Autodesk Inventor part; units mm, degrees
ref_plane "YZ Plane" through (0, 0, 0) normal (1, 0, 0) x (0, 1, 0)
ref_plane "XZ Plane" through (0, 0, 0) normal (0, 1, 0) x (-1, 0, 0)
ref_plane "XY Plane" through (0, 0, 0) normal (0, 0, 1) x (1, 0, 0)
sketch "スケッチ1" plane through (0, 0, 0) normal (0, 0, 1) x (1, 0, 0)
  circle A0 centre (0, 0) radius 1.5
  dimension "d0" = 3
extrude "押し出し1" add sketch "スケッチ1" along normal blind 6
sketch "スケッチ2" plane through (0, 0, 6) normal (0, 0, 1) x (1, 0, 0)
  circle A0 centre (0, 0) radius 1.5
  circle A1 centre (0, 0) radius 3
  dimension "d3" = 6
extrude "押し出し2" add sketch "スケッチ2" along normal blind 2 contours A0 | A1
fillet "フィレット1" radius 2 1 edges at (-3, 0, 8)
thread "ねじ1"
sketch "スケッチ3" plane through (0, 0, 0) normal (0, 0, -1) x (-1, 0, 0)
  circle A0 centre (0, 0) radius 1.5
extrude "押し出し3" add sketch "スケッチ3" along normal blind 9
sketch "スケッチ4" plane through (0, 0, -9) normal (0, 0, -1) x (-1, 0, 0)
  circle A0 centre (0, 0) radius 1.5
extrude "押し出し4" add sketch "スケッチ4" along normal blind 7
properties part number "SB　22mmなべネジ" material "Steel, Mild"
The model under review builds one solid part; all positions refer to its coordinate system, in mm. A direction names the side the tool comes from. Give positions to 0.01 mm unless a question says otherwise; leave off trailing zeros. Loops run counter-clockwise (first coordinate to the right, second up) from the corner with the lowest first, then second, coordinate; pieces in that order, holes last. Notation, with made-up numbers: (83.25, 38) -> (136.25, 38) arc R10 ccw to (136.25, 42) -> close; hole circle Ø11 at (55, -5.75). An arc over 180 degrees is marked (long way). Answer as a JSON object with one key per item and string values. Group by question number.
Q1. Wall thickness on line 1 along Z through (x, y) = (-0.5, 1); line 2 along X through (y, z) = (0, 1.25): over which ranges is each line inside the solid? List them lowest first.
Q2. Tool access review of faces 1 (the flat face through (1.3, -1.3, 6)), 2 (the flat face through (0, 0, -16)): name each direction out of +Z, -Z, +X, -X, +Y, -Y from which nothing blocks a thin tool from reaching the whole face with its end or side.
Q3. Insertion check: pin 1 (3 mm diameter, centred on y = 0.5, z = -9.5, fed in from -X); pin 2 (1.5 mm diameter, centred on x = 2.5, y = -1, fed in from +Z); pin 3 (1 mm diameter, centred on x = -1.5, y = 0, fed in from +Z). Each pin has a flat end and moves straight along its axis. Give the tip position at first contact, or say it passes through.
Q4. Take a section at A-A (z = -5). Write out the cut boundary in (x, y).
Answer below:
{
 "1": {"line 1": "z = -16 to 8", "line 2": "x = -1.5 to 1.5"},
 "2": {"face 1": "-Z", "face 2": "-Z, +X, -X, +Y, -Y"},
 "3": {"pin 1": "stops at x = -1.5", "pin 2": "stops at z = 7.76", "pin 3": "stops at z = 8"},
 "4": {"outline": "circle Ø3 at (0, 0)"}
}
